from build123d import *

# Parameters (mm, degrees)
ESQUISSE1_R        = 4
BOSS_EXTRU_1_DEPTH = 815
CONG_1_R           = 3


with BuildPart() as part:
    # Esquisse1 → Boss.-Extru.1 (new body)
    with BuildSketch(Plane(origin=(1000, 0, 0), x_dir=(0, 0, -1), z_dir=(1, 0, 0))):
        Polygon((22.5, -4), (12.5, -4), (12.5, 4), (22.5, 4), (22.5, 22.5), (4, 22.5), (4, 12.5), (-4, 12.5), (-4, 22.5), (-22.5, 22.5), (-22.5, 4), (-12.5, 4), (-12.5, -4), (-22.5, -4), (-22.5, -22.5), (-4, -22.5), (-4, -12.5), (4, -12.5), (4, -22.5), (22.5, -22.5), align=None)
        Circle(ESQUISSE1_R, mode=Mode.SUBTRACT)
    extrude(amount=-BOSS_EXTRU_1_DEPTH)

    # Congé1
    cong_1_edges = [part.edges().sort_by_distance(p)[0] for p in [
        (592.5, -22.5, -22.5),
        (592.5, -22.5, 22.5),
        (592.5, 22.5, 22.5),
        (592.5, 22.5, -22.5),
    ]]
    fillet(cong_1_edges, radius=CONG_1_R)


solid = part.part
Could you check a few things on this model? Use its own coordinates, in mm. Give positions to 0.01 mm unless a question says otherwise; leave off trailing zeros. Order: outer loops, then holes, each group sorted by start corner. A loop starts at its lowest first (then second) coordinate and runs counter-clockwise, first axis right, second up. Notation, with made-up numbers: (9.5, 86) - (33.5, 86) arc R8 cw to (33.5, 94) - close; hole circle Ø10 at (82, 29). An arc over 180 degrees is marked (long way). One line per question, with ' | ' between items. Start each with the question number.
Item 1: I want a section at A-A on x = 292. Write out the boundary of the cut face in (y, z).
Item 2: I'm going to push flat-ended pins straight in: pin 1 Ø4 at (x, y) = (588.5, -1) entering from +Z; pin 2 Ø2.5 at (x, z) = (400.5, -1) entering from +Y; pin 3 Ø6.5 at (x, y) = (500.5, 1.5) entering from -Z. Where does each tip first touch, or does it pass through?
Item 3: I need wall thicknesses on probe 1 along Z at (x, y) = (896, -16); probe 2 along Y at (x, z) = (790.5, 0). Which ranges of each line are inside material? Lowest first, please. Write a range as [from, to].
Verdict:
1) outline: (-22.5, -19.5) arc R3 ccw to (-19.5, -22.5) - (-4, -22.5) - (-4, -12.5) - (4, -12.5) - (4, -22.5) - (19.5, -22.5) arc R3 ccw to (22.5, -19.5) - (22.5, -4) - (12.5, -4) - (12.5, 4) - (22.5, 4) - (22.5, 19.5) arc R3 ccw to (19.5, 22.5) - (4, 22.5) - (4, 12.5) - (-4, 12.5) - (-4, 22.5) - (-19.5, 22.5) arc R3 ccw to (-22.5, 19.5) - (-22.5, 4) - (-12.5, 4) - (-12.5, -4) - (-22.5, -4) - close; hole circle Ø8 at (0, 0)
2) pin 1: z = 12.5 | pin 2: y = 12.5 | pin 3: z = -22.5
3) probe 1: [-22.5, -4], [4, 22.5] | probe 2: [-12.5, -4], [4, 12.5]
